Model file for the job. Use its own axes, mm. A direction names the side the tool comes from. Round coordinates to 2 decimals unless told otherwise and drop trailing zeros. Order: outer loops, then holes, each group sorted by start corner. A loop starts at its lowest first (then second) coordinate and runs counter-clockwise, first axis right, second up. Notation, with made-up numbers: (14.5, 76.5) -> (47.5, 76.5) arc R34 cw to (47.5, 108.5) -> close; hole circle Ø6 at (-2.5, 79). An arc over 180 degrees is marked (long way). Use CSV: the item, a comma, the result in double quotes.
```python
from build123d import *

# Parameters (mm, degrees)
SKIZZE1_W                       = 16.1
SKIZZE1_H                       = 120
AUFSATZ_LINEAR_AUSTRAGEN1_DEPTH = 17.6
AUFSATZ_LINEAR_AUSTRAGEN2_DEPTH = 1.85
SKIZZE3_R                       = 1.05
SCHNITT_LINEAR_AUSTRAGEN1_DEPTH = 13
SKIZZE4_R                       = 1.05
SKIZZE4_W                       = 12.4
SKIZZE4_H                       = 23.5
SCHNITT_LINEAR_AUSTRAGEN2_DEPTH = 65.807291256
SCHNITT_LINEAR_AUSTRAGEN3_DEPTH = 67.29021421


with BuildPart() as part:
    # Skizze1 → Aufsatz-Linear austragen1 (new body)
    with BuildSketch(Plane(origin=(0, 0, 0), x_dir=(1, 0, 0), z_dir=(0, 1, 0))):
        Rectangle(SKIZZE1_W, SKIZZE1_H)
    extrude(amount=AUFSATZ_LINEAR_AUSTRAGEN1_DEPTH)

    # Skizze2 → Aufsatz-Linear austragen2 (add)
    with BuildSketch(Plane.XY.offset(60)):
        Polygon((0, 17.5), (-7.95, 0), (7.95, 0), align=None)
    extrude(amount=AUFSATZ_LINEAR_AUSTRAGEN2_DEPTH)

    # Skizze3 → Schnitt-Linear austragen1 (cut)
    with BuildSketch(Plane.XY.offset(61.85)):
        with Locations((0, 4.89)):
            Circle(SKIZZE3_R)
    extrude(amount=-SCHNITT_LINEAR_AUSTRAGEN1_DEPTH, mode=Mode.SUBTRACT)

    # Skizze4 → Schnitt-Linear austragen2 (cut, through all)
    with BuildSketch(Plane(origin=(0, 17.6, 0), x_dir=(1, 0, 0), z_dir=(0, 1, 0))):
        with Locations(Location((0, 58.1, 0), (0, 0, 270))):
            Circle(SKIZZE4_R)
        with Locations(Location((0, 29.9, 0), (0, 0, 270))):
            Circle(SKIZZE4_R)
        with Locations((0, 44)):
            Rectangle(SKIZZE4_W, SKIZZE4_H)
    extrude(amount=-SCHNITT_LINEAR_AUSTRAGEN2_DEPTH, mode=Mode.SUBTRACT)

    # Skizze5 → Schnitt-Linear austragen3 (cut, through all)
    with BuildSketch(Plane(origin=(8.05, 0, 0), x_dir=(0, 0, -1), z_dir=(1, 0, 0))):
        with BuildLine():
            Line((60, 11.6), (31, 11.6))
            ThreePointArc((31, 11.6), (24.636038969, 8.963961031), (22, 2.6))
            Line((22, 2.6), (22, 0))
            Line((22, 0), (60, 0))
            Line((60, 0), (60, 11.6))
        make_face()
    extrude(amount=-SCHNITT_LINEAR_AUSTRAGEN3_DEPTH, mode=Mode.SUBTRACT)


solid = part.part
```
Q1. Cut at A-A (y = 14). Give the cut face in (x, z).
From the geometry:
outline,"(-8.05, -60) -> (8.05, -60) -> (8.05, 60) -> (1.59, 60) -> (1.59, 61.85) -> (-1.59, 61.85) -> (-1.59, 60) -> (-8.05, 60) -> close; hole (-6.2, -55.75) -> (6.2, -55.75) -> (6.2, -32.25) -> (-6.2, -32.25) -> close; hole circle Ø2.1 at (0, -58.1); hole circle Ø2.1 at (0, -29.9)"
Q2. Cut at C-C (x = 2.75). Give the cut face in (y, z), plus the area to 3 significant figures.
From the geometry:
outline,"(0, -22) -> (2.6, -22) arc R9 cw to (11.6, -31) -> (11.6, -32.25) -> (17.6, -32.25) -> (17.6, 60) -> (11.45, 60) -> (11.45, 61.85) -> (0, 61.85) -> close; (11.6, -60) -> (17.6, -60) -> (17.6, -55.75) -> (11.6, -55.75) -> close"
area,"1,570 mm²"
Q3. Cut at B-B (z = -58.1). Give the cut face in (x, y).
From the geometry:
outline,"(-8.05, 11.6) -> (-1.05, 11.6) -> (-1.05, 17.6) -> (-8.05, 17.6) -> close; (1.05, 11.6) -> (8.05, 11.6) -> (8.05, 17.6) -> (1.05, 17.6) -> close"
Q4. Cut at D-D (y = 4.89). Give the cut face in (x, z).
From the geometry:
outline,"(-8.05, -22.3) -> (8.05, -22.3) -> (8.05, 60) -> (5.73, 60) -> (5.73, 61.85) -> (1.05, 61.85) -> (1.05, 48.85) -> (-1.05, 48.85) -> (-1.05, 61.85) -> (-5.73, 61.85) -> (-5.73, 60) -> (-8.05, 60) -> close"
Q5. Mould opens along Y. For faces 4 (the cylindrical face through (-0.228, 3.865, 55.441)), 5 (the flat face through (-7, 11.6, -48)), 6 (the flat face through (0, 17.6, 12)), 7 (the flat face through (0, 5, 48.85)) say: +Y half, -Y half, draft (parallel to the pull), parting line (faces both ways), or undercut.
From the geometry:
face 4,"undercut"
face 5,"-Y half"
face 6,"+Y half"
face 7,"undercut"
Q6. Probe line 1 along Y through (x, z) = (0, 56); line 2 along X through (y, z) = (15.75, -58.1); line 3 along Z through (x, y) = (-6, 14.25). List the from-to ranges inside material, lowest first.
From the geometry:
line 1,"y = 0 to 3.84, 5.94 to 17.6"
line 2,"x = -8.05 to -1.05, 1.05 to 8.05"
line 3,"z = -60 to -55.75, -32.25 to 60"
Q7. Pin check, flat tips, straight feed: pin 1 (3.5 mm diameter, centred on x = 0, z = -29.9, fed in from -Y); pin 2 (1.3 mm diameter, centred on x = 0, y = 0.5, fed in from -Z); pin 3 (1.9 mm diameter, centred on x = 0, y = 4.89, fed in from +Z). Stop position of each tip, or through.
From the geometry:
pin 1,"stops at y = 11.14"
pin 2,"stops at z = -22"
pin 3,"stops at z = 48.85"
Q8. Which spindle directions (+Z, -Z, +X, -X, +Y, -Y) get a long thin tool onto all of the face, cutting with end or side? Do faces 1 (the flat face through (0, 1, -22)), 2 (the flat face through (4.03, 8.63, 60.91)), 3 (the flat face through (6.2, 15, -44)). Say none if no direction does.
From the geometry:
face 1,"-Z, +X, -X, -Y"
face 2,"+Z, +X, +Y"
face 3,"+Y, -Y"
